```python
from build123d import *

# Parameters (mm, degrees)
F1_DEPTH = 80
F2_W     = 30
F2_H     = 30
F3_DEPTH = 8
F4_W     = 30
F4_H     = 30
F5_DEPTH = 8


with BuildPart() as f1:
    # F0 (on Front) → F1 (new body)
    with BuildSketch(Plane.XZ):
        Polygon((-62.069241, -21.991899), (-62.35861, -41.958228), (64.962916, -41.958228), (64.962916, 17.362025), (26.477087, 17.362025), align=None)
    extrude(amount=F1_DEPTH)

    # F2 (on face) → F3 (cut)
    with BuildSketch(Plane.XY.offset(17.362025)):
        with Locations((46.655876, -60.924847)):
            Rectangle(F2_W, F2_H)
    extrude(amount=-F3_DEPTH, mode=Mode.SUBTRACT)

    # F4 (on face) → F5 (cut)
    with BuildSketch(Plane(origin=(-2.076283, 0, 4.671638), x_dir=(0.913812, 0, 0.406138), z_dir=(-0.406138, 0, 0.913812))):
        with Locations((-27.1411, -60.458847)):
            Rectangle(F4_W, F4_H)
    extrude(amount=-F5_DEPTH, mode=Mode.SUBTRACT)


solid = f1.part
```
Can you work these out from the model? Positions are in its coordinate system, mm. A direction names the side the tool comes from. Coordinates: 2 decimals unless noted, no trailing zeros. Write each loop counter-clockwise with the first axis right and the second up, starting at its lowest first coordinate (ties: lowest second). Pieces come first, ordered by that corner, then holes. Notation, with made-up numbers: M -38.75,51 L -25.75,51 A26 cw -25.75,74 Z; hole C -33.75,64.25 d5. An arc over 180 degrees is marked long. Write item = value, one per line. Start each with the question number.
Q1. If we section it at D-D, the plane z = -4: Write out the boundary of the cut face in (x, y), then the cut area to 3 significant figures.
Q2. If we section it at A-A, the plane x = 56.5: Write out the boundary of the cut face in (y, z).
Q3. If we section it at B-B, the plane y = -66: Write out the boundary of the cut face in (x, z).
Q4. I'm going to push flat-ended pins straight in: pin 1 (8 mm diameter, centred on x = -26.5, y = -27, fed in from +Z); pin 2 (9 mm diameter, centred on y = -63.5, z = 12.5, fed in from -X); pin 3 (2 mm diameter, centred on y = -71.5, z = 5, fed in from -X). Where does each tip first touch, or does it pass through?
Q5. If I drill on L1, parallel to Y at x = -19.5, z = -3.5; L2, parallel to X at y = -50, z = -14; L3, parallel to Z at x = 53, y = -59, over which ranges is the centre line in solid material (lowest first)? Write a range as [from, to].
Q6. On a 3-axis mill with a long thin cutter (end or side, diameter ignored), from which of +Z, -Z, +X, -X, +Y, -Y can I reach the whole of each face in a straight line? I mean faces 4 (the face through (-11.57, -60.67, -3.86)), 5 (the face through (64.963, -39, -13)), 6 (the face through (46, -75.925, 13)). Say none if no direction works.
Q7. If we section it at C-C, the plane z = -16: Write out the boundary of the cut face in (x, y), then the cut area to 3 significant figures.
Q8. Thinking about a two-plate mould opening in Y: for faces 1 (the face through (-17.18, -39.44, -2.04)), 2 (the face through (-38.984, -60.669, -16.048)), 3 (the face through (15, -80, -18)), which applies, released by +Y, released by -Y, zero draft, split by the parting line, or undercut?
Check sheet entries:
q1.outline = M -21.59,-80 L 64.96,-80 L 64.96,0 L -21.59,0 L -21.59,-45.46 L -11.51,-45.46 L -11.51,-75.46 L -21.59,-75.46 Z
q1.area = 6,620 mm²
q2.outline = M -80,-41.96 L 0,-41.96 L 0,17.36 L -45.92,17.36 L -45.92,9.36 L -75.92,9.36 L -75.92,17.36 L -80,17.36 Z
q3.outline = M -62.36,-41.96 L 64.96,-41.96 L 64.96,17.36 L 61.66,17.36 L 61.66,9.36 L 31.66,9.36 L 31.66,17.36 L 26.48,17.36 L -13.17,-0.26 L -9.92,-7.57 L -37.34,-19.75 L -40.59,-12.44 L -62.07,-21.99 Z
q4.pin_1 = -4.41
q4.pin_2 = 5.41
q4.pin_3 = -3.59
q5.L1 = [-80, -75.46], [-45.46, 0]
q5.L2 = [-44.09, -39.89], [-24.39, 64.96]
q5.L3 = [-41.96, 9.36]
q6.face_4 = -X
q6.face_5 = +Z, -Z, +X, +Y, -Y
q6.face_6 = +Z
q7.outline = M -48.59,-80 L 64.96,-80 L 64.96,0 L -48.59,0 Z; hole M -39,-75.46 L -28.89,-75.46 L -28.89,-45.46 L -39,-45.46 Z
q7.area = 8,780 mm²
q8.face_1 = zero draft
q8.face_2 = undercut
q8.face_3 = released by -Y
